Can you work these out from the drawing? Everything is in mm from the part's minimum corner. A direction names the side the tool comes from. Coordinates: 2 decimals unless noted, no trailing zeros. Order: outer loops, then holes, each group sorted by start corner. A loop starts at its lowest first (then second) coordinate and runs counter-clockwise, first axis right, second up. Notation, with made-up numbers: M -35,67.25 L 2,67.25 A23 ccw 2,82.25 Z; hole C 11,23 d7. An arc over 180 degrees is marked long. One line per question, with ' | ' between items. Start each with the question number.
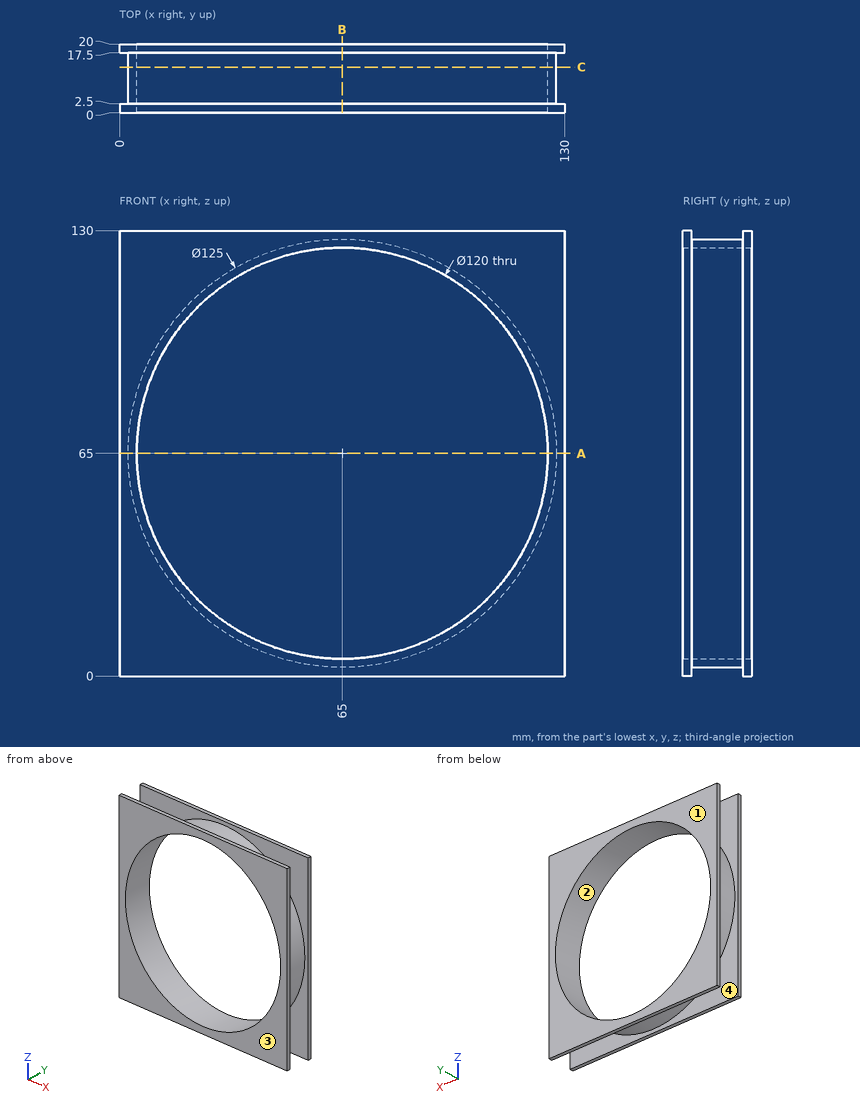
(1) For P1, Ø5, axis at y = 10.5, z = 20.5, coming from the +X side; P2, Ø3, axis at x = 47.5, y = 12, coming from the +Z side; P3, Ø1.5, axis at y = 9.5, z = 87, coming from the +X side, each with a flat end and sliding along its axis, tell me the tip position at first contact or that it passes through.
(2) Imagine slicing it at B-B, the plane x = 65. Write out the boundary of the cut face in (y, z).
(3) Imagine slicing it at A-A, the plane z = 65. Write out the boundary of the cut face in (x, y).
(4) We'd pull the mould along Z, two halves only. Please class the marked faces 1 and 2: +Z half, -Z half, draft (parallel to the pull), parting line (faces both ways), or undercut.
(5) Imagine slicing it at C-C, the plane y = 13.25. Write out the boundary of the cut face in (x, z), plus the area to 3 significant figures.
(6) If I drill on line 1 along Z through (x, y) = (65, 12); line 2 along Y through (x, z) = (104.5, 11), over which ranges is the centre line in solid material (lowest first)? Write a range as from..to.
(7) On a 3-axis mill with a long thin cutter (end or side, diameter ignored), from which of +Z, -Z, +X, -X, +Y, -Y can I reach the whole of each face in a straight line? I mean the marked faces 3 and 4. Say none if no direction works.
Answers:
1) P1: x = 111.28 | P2: z = 125.42 | P3: x = 123.78
2) outline: M 0,0 L 2.5,0 L 2.5,2.5 L 17.5,2.5 L 17.5,0 L 20,0 L 20,5 L 0,5 Z; M 0,125 L 20,125 L 20,130 L 17.5,130 L 17.5,127.5 L 2.5,127.5 L 2.5,130 L 0,130 Z
3) outline: M 0,0 L 5,0 L 5,20 L 0,20 L 0,17.5 L 2.5,17.5 L 2.5,2.5 L 0,2.5 Z; M 125,0 L 130,0 L 130,2.5 L 127.5,2.5 L 127.5,17.5 L 130,17.5 L 130,20 L 125,20 Z
4) face 1: draft | face 2: undercut
5) outline: C 65,65 d125; hole C 65,65 d120 | area: 962 mm²
6) line 1: 2.5..5, 125..127.5 | line 2: 0..2.5, 17.5..20
7) face 3: +Z, -Z, +X, -X, -Y | face 4: none
